Verification items for this drawing (mm, ordinates from the low corner). Round coordinates to 2 decimals unless told otherwise and drop trailing zeros. Loops run counter-clockwise (first coordinate to the right, second up) from the corner with the lowest first, then second, coordinate; pieces in that order, holes last. Notation, with made-up numbers: (77, 2.5) -> (129, 2.5) arc R9 cw to (129, 16.5) -> close; hole circle Ø1 at (-27, 66.25). An arc over 180 degrees is marked (long way). One line per question, with ' | ' between items.
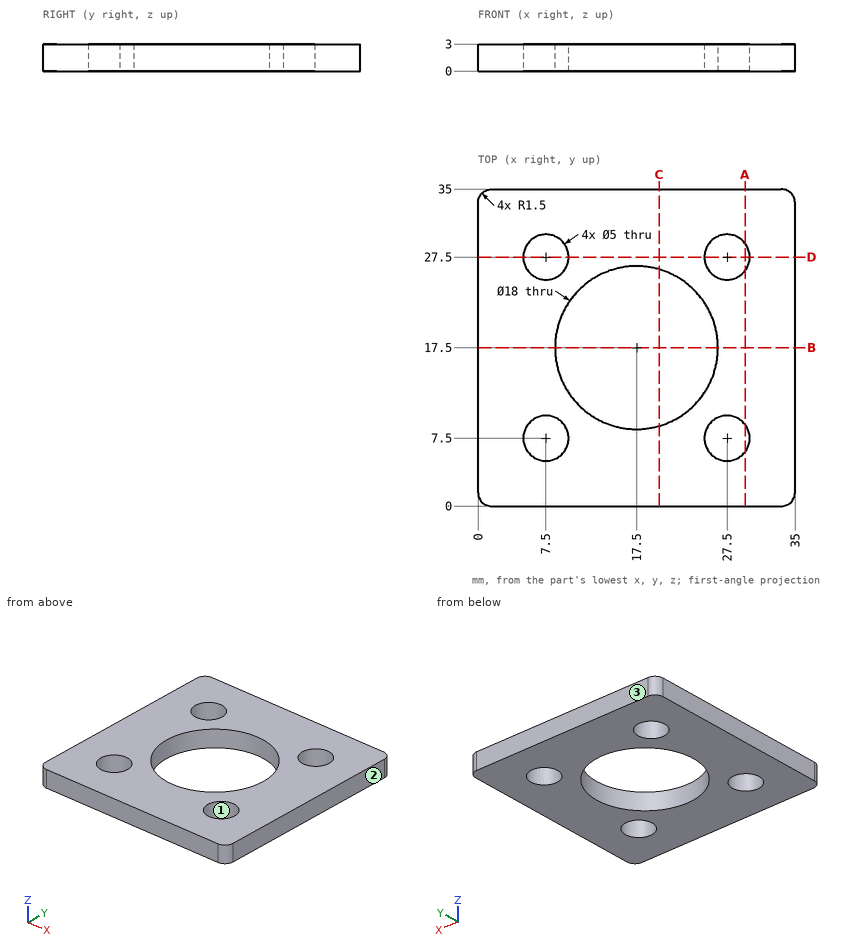
(1) Sectioned sample at C-C, the plane x = 20. Record the cut outline in (y, z), and give its area (3 significant figures).
Answer:
outline: (0, 0) -> (8.85, 0) -> (8.85, 3) -> (0, 3) -> close; (26.15, 0) -> (35, 0) -> (35, 3) -> (26.15, 3) -> close | area: 53.1 mm2
(2) Mould release check, pull along X, two halves, no side actions. Record for the marked faces 1, 2 and 3: +X half, -X half, draft (parallel to the pull), parting line (faces both ways), or undercut.
Answer:
face 1: undercut | face 2: +X half | face 3: draft
(3) Sectioned sample at A-A, the plane x = 29.5. Record the cut outline in (y, z).
Answer:
outline: (0, 0) -> (6, 0) -> (6, 3) -> (0, 3) -> close; (9, 0) -> (26, 0) -> (26, 3) -> (9, 3) -> close; (29, 0) -> (35, 0) -> (35, 3) -> (29, 3) -> close
(4) Sectioned sample at B-B, the plane y = 17.5. Record the cut outline in (x, z), and give its area (3 significant figures).
Answer:
outline: (0, 0) -> (8.5, 0) -> (8.5, 3) -> (0, 3) -> close; (26.5, 0) -> (35, 0) -> (35, 3) -> (26.5, 3) -> close | area: 51.0 mm2
(5) Sectioned sample at D-D, the plane y = 27.5. Record the cut outline in (x, z), and give its area (3 significant figures).
Answer:
outline: (0, 0) -> (5, 0) -> (5, 3) -> (0, 3) -> close; (10, 0) -> (25, 0) -> (25, 3) -> (10, 3) -> close; (30, 0) -> (35, 0) -> (35, 3) -> (30, 3) -> close | area: 75.0 mm2
(6) Go/stop test with a flat-tipped pin: pin 1 (3 mm diameter, centred on x = 27.5, y = 27.5, fed in from +Z). Record where the tip stops, or that it passes through.
Answer:
pin 1: passes through
(7) Scan lines: probe 1 along Y at (x, z) = (27.5, 1.9); probe 2 along X at (y, z) = (25.5, 1.95); probe 3 along Y at (x, z) = (12, 1.05). Record each from-to range of solid material in increasing order.
Answer:
probe 1: y = 0 to 5, 10 to 25, 30 to 35 | probe 2: x = 0 to 6, 9 to 13.38, 21.62 to 26, 29 to 35 | probe 3: y = 0 to 10.38, 24.62 to 35
